Work out the finished part from the listing and answer in its coordinate system (mm). A direction names the side the tool comes from. Round coordinates to 2 decimals unless told otherwise and drop trailing zeros. Loops run counter-clockwise (first coordinate to the right, second up) from the corner with the lowest first, then second, coordinate; pieces in that order, holes last. Notation, with made-up numbers: (-28, 6.5) - (28, 6.5) arc R31 ccw to (28, 35.5) - close; hole circle Ø1 at (20.25, 71). An arc over 180 degrees is marked (long way). Answer as CSV lines item,"result". Start each with the question number.
Q1. Section D-D on y = 0.55 is taken. Write down the section's boundary in (x, z).
Q2. Straight lines are drawn through the part: L1, parallel to X at y = 4.15, z = 7.5; L2, parallel to X at y = 1.1, z = 18.4; L3, parallel to Y at x = -17, z = -6.5. For each, find the intervals that lie inside material, in ascending order. Write a range as [from, to].
Q3. Each of these flat-tipped pins is pushed along its axis until it touches: pin 1 Ø3 at (x, z) = (0, 18.4) entering from +Y; pin 2 Ø1.1 at (y, z) = (4.5, 3) entering from +X; pin 3 Ø0.8 at (x, y) = (2, 4.5) entering from +Z; pin 4 Ø0.8 at (x, y) = (7, 4.5) entering from -Z. Where does it stop, or does it pass through?
Q4. Section C-C on z = -4 is taken. Write down the section's boundary in (x, y).
Q5. Section A-A on z = -9.2 is taken. Write down the section's boundary in (x, y), then the cut area to 3 significant figures.
Q6. The mould has two halves that part along X. Classify faces 1 (the face through (15.532, 3.274, -13.586)), 2 (the face through (-13.248, 4.5, 6)), 3 (the face through (-11.7, 4.5, 0.5)), 4 (the face through (-0.1, 3.3, 14.4)): +X half, -X half, draft (parallel to the pull), parting line (faces both ways), or undercut.
Q7. Section B-B on y = 3.25 is taken. Write down the section's boundary in (x, z), then the cut area to 3 significant figures.
Q8. For faces 5 (the face through (11.3, 4.5, -0.5)), 6 (the face through (-4, 3, 20)), 7 (the face through (3.2, 4.5, -11.137)), determine the directions among +Z, -Z, +X, -X, +Y, -Y from which every point of the face is accessible in a straight line to the end or side of a thin tool.
```python
from build123d import *

# Parameters (mm, degrees)
SKETCH1_R               = 22.5
PLATE_DEPTH             = 5
OPENING_START           = 1.5
OPENING_FOR_SCREW_DEPTH = 5
SKETCH7_R               = 1.75
SCREW_HOLE_DEPTH        = 5
CIRPATTERN20_COUNT      = 3
SKETCH10_W              = 45
SKETCH10_H              = 1
SKETCH10_W_2            = 1
SKETCH10_H_2            = 45
CUT_EXTRUDE5_DEPTH      = 1
CUT_EXTRUDE6_DEPTH      = 1


with BuildPart() as part:
    # Sketch1 → plate (new body)
    with BuildSketch(Plane(origin=(0, 0, 0), x_dir=(1, 0, 0), z_dir=(0, 1, 0))):
        Circle(SKETCH1_R)
    extrude(amount=PLATE_DEPTH)

    # Sketch6 → opening for screw (cut)
    with BuildSketch(Plane(origin=(0, 5, 0), x_dir=(1, 0, 0), z_dir=(0, 1, 0)).offset(OPENING_START)):
        with BuildLine():
            Line((-4, -22.5), (-4, -18.4))
            ThreePointArc((-4, -18.4), (0, -14.4), (4, -18.4))
            Line((4, -18.4), (4, -22.5))
            ThreePointArc((4, -22.5), (0, -26.5), (-4, -22.5))
        make_face()
    opening_for_screw = extrude(amount=-OPENING_FOR_SCREW_DEPTH, mode=Mode.SUBTRACT)

    # Sketch7 → screw hole (cut)
    with BuildSketch(Plane(origin=(0, 1.5, 0), x_dir=(1, 0, 0), z_dir=(0, 1, 0))):
        with Locations((0, -18.4)):
            Circle(SKETCH7_R)
    screw_hole = extrude(amount=-SCREW_HOLE_DEPTH, mode=Mode.SUBTRACT)

    # CirPattern20: opening for screw, screw hole ×3 about axis
    cirpattern20_axis = Axis((0, 0, 0), (0, 1, 0))
    for i in range(1, CIRPATTERN20_COUNT):
        add(opening_for_screw.rotate(cirpattern20_axis, i * 360 / CIRPATTERN20_COUNT), mode=Mode.SUBTRACT)
        add(screw_hole.rotate(cirpattern20_axis, i * 360 / CIRPATTERN20_COUNT), mode=Mode.SUBTRACT)

    # Sketch10 → Cut-Extrude5 (cut)
    with BuildSketch(Plane(origin=(0, 5, 0), x_dir=(1, 0, 0), z_dir=(0, 1, 0))):
        Rectangle(SKETCH10_W, SKETCH10_H)
        Rectangle(SKETCH10_W_2, SKETCH10_H_2)
    extrude(amount=-CUT_EXTRUDE5_DEPTH, mode=Mode.SUBTRACT)

    # Sketch11 → Cut-Extrude6 (cut)
    with BuildSketch(Plane(origin=(0, 5, 0), x_dir=(1, 0, 0), z_dir=(0, 1, 0))):
        Polygon((2.616666667, 13.742425761), (2.616666667, 15.289220632), (3.675, 15.289220632), (3.675, 13.742425761), (5.303205128, 13.742425761), (5.303205128, 12.684092427), (3.675, 12.684092427), (3.675, 11.137297556), (2.616666667, 11.137297556), (2.616666667, 12.684092427), (0.988461538, 12.684092427), (0.988461538, 13.742425761), align=None)
        Polygon((6.136388221, 16.510374479), (7.479657452, 16.510374479), (8.806390224, 14.471301963), (10.135667067, 16.510374479), (11.480208333, 16.510374479), (9.47802484, 13.43968137), (11.6125, 10.160374479), (10.269230769, 10.160374479), (8.806390224, 12.409332812), (7.339733574, 10.160374479), (5.995192308, 10.160374479), (8.134755609, 13.440953405), align=None)
        Polygon((-18.458103671, -3.794817635), (-18.458103671, -2.248022763), (-17.399770338, -2.248022763), (-17.399770338, -3.794817635), (-15.771565209, -3.794817635), (-15.771565209, -4.853150968), (-17.399770338, -4.853150968), (-17.399770338, -6.39994584), (-18.458103671, -6.39994584), (-18.458103671, -4.853150968), (-20.086308799, -4.853150968), (-20.086308799, -3.794817635), align=None)
        Polygon((-15.07957803, -1.026868917), (-13.811358879, -1.026868917), (-12.677975466, -3.254202651), (-11.544592052, -1.026868917), (-10.276372902, -1.026868917), (-12.108103671, -4.626728693), (-12.108103671, -7.376868917), (-13.247847261, -7.376868917), (-13.247847261, -4.626728693), align=None)
    extrude(amount=-CUT_EXTRUDE6_DEPTH, mode=Mode.SUBTRACT)


solid = part.part
```
Findings:
1,outline,"circle Ø45 at (0, 0); hole circle Ø3.5 at (-15.93, -9.2); hole circle Ø3.5 at (0, 18.4); hole circle Ø3.5 at (15.93, -9.2)"
2,L1,"x = [-21.21, -0.5], [0.5, 21.21]"
2,L2,"x = [-12.95, -1.75], [1.75, 12.95]"
2,L3,"y = [0, 1.5]"
3,pin 1,"passes through"
3,pin 2,"stops at x = 22.37"
3,pin 3,"stops at z = 15.2"
3,pin 4,"stops at z = -21.51"
4,outline,"(-22.14, 0) - (22.14, 0) - (22.14, 5) - (0.5, 5) - (0.5, 4) - (-0.5, 4) - (-0.5, 5) - (-22.14, 5) - close"
5,outline,"(-20.53, 0) - (-17.68, 0) - (-17.68, 1.5) - (-20.53, 1.5) - close; (-14.18, 0) - (14.18, 0) - (14.18, 1.5) - (11.93, 1.5) - (11.93, 5) - (0.5, 5) - (0.5, 4) - (-0.5, 4) - (-0.5, 5) - (-11.93, 5) - (-11.93, 1.5) - (-14.18, 1.5) - close; (17.68, 0) - (20.53, 0) - (20.53, 1.5) - (17.68, 1.5) - close"
5,area,"134 mm^2"
6,face 1,"+X half"
6,face 2,"undercut"
6,face 3,"draft"
6,face 4,"undercut"
7,outline,"(-21.18, -7.61) - (-17.93, -5.74) arc R4 cw to (-13.93, -12.66) - (-17.18, -14.53) arc R22.5 ccw to (17.18, -14.53) - (13.93, -12.66) arc R4 cw to (17.93, -5.74) - (21.18, -7.61) arc R22.5 ccw to (4, 22.14) - (4, 18.4) arc R4 cw to (-4, 18.4) - (-4, 22.14) arc R22.5 ccw to start"
7,area,"1,420 mm^2"
8,face 5,"+X, -X, +Y"
8,face 6,"+Z, +Y"
8,face 7,"+Y"
